```python
from build123d import *

# Parameters (mm, degrees)
SKETCH001_R       = 1.687519
PAD001_DEPTH      = 1.5
SKETCH_R          = 1.746092
PAD_DEPTH         = 2
FUSION_ROLL_ANGLE = 90


with BuildPart() as base_and_horizontal_holder:
    # Sketch001 → Pad001 (new body)
    with BuildSketch(Plane.XZ.offset(1.2525)):
        with BuildLine():
            Line((10.979984, 0), (69.999984, 0))
            Line((69.999984, 0), (69.999984, -21.282469))
            ThreePointArc((66.378106, -24.904346), (68.93916, -23.843523), (69.999984, -21.282469))
            Line((22.859289, -24.904346), (66.378106, -24.904346))
            ThreePointArc((10.979984, -13.025041), (14.459352, -21.424978), (22.859289, -24.904346))
            Line((10.979984, 0), (10.979984, -13.025041))
        make_face()
        with Locations((67.250752, -3.727469)):
            Circle(SKETCH001_R, mode=Mode.SUBTRACT)
        with Locations((16.457752, -18.999969)):
            Circle(SKETCH001_R, mode=Mode.SUBTRACT)
    extrude(amount=-PAD001_DEPTH)


with BuildPart() as obj1:
    # Sketch → Pad (new body)
    with BuildSketch(Plane.XY):
        with BuildLine():
            Line((11.012519, -1.25328), (11.012519, 6.997142))
            ThreePointArc((13.001287, 8.992943), (11.59459, 8.405902), (11.012519, 6.997142))
            Line((13.001287, 8.992943), (15, 9))
            ThreePointArc((16.997615, 7.009425), (16.412099, 8.419465), (15, 9))
            Line((16.997615, 7.009425), (16.997615, 4))
            ThreePointArc((16.997615, 4), (17.290509, 3.292893), (17.997615, 3))
            Line((17.997615, 3), (62, 3))
            Line((62, 3), (62.401287, 3))
            ThreePointArc((62.401287, 3), (64.238855, 3.761145), (65, 5.598713))
            Line((65, 5.598713), (65, 6))
            Line((65, 6), (62, 10))
            ThreePointArc((65, 13), (62.87868, 12.12132), (62, 10))
            Line((65, 13), (67, 13))
            ThreePointArc((70, 10), (69.12132, 12.12132), (67, 13))
            Line((70, 10), (70, -1.25328))
            Line((11.012519, -1.25328), (70, -1.25328))
        make_face()
        with Locations((13.988471, 5.299093)):
            Circle(SKETCH_R, mode=Mode.SUBTRACT)
        with Locations((66.082271, 10.342403)):
            Circle(SKETCH_R, mode=Mode.SUBTRACT)
    extrude(amount=PAD_DEPTH)

    # Fusion: union base_and_horizontal_holder
    add(base_and_horizontal_holder.part)


with BuildPart() as obj1_1:
    # Fusion roll: moved
    add(obj1.part.rotate(Axis((0, 0, 0), (1, 0, 0)), FUSION_ROLL_ANGLE))


with BuildPart() as obj1_2:
    # Fusion placement: moved
    add(obj1_1.part.moved(Location((-10.98, 2, 1.25))))


solid = obj1_2.part
```
Input: part model. Units: mm. Frame: model coordinates. A direction names the side the tool comes from. Coordinates: 2 decimals unless noted, no trailing zeros. Write each loop counter-clockwise with the first axis right and the second up, starting at its lowest first coordinate (ties: lowest second). Pieces come first, ordered by that corner, then holes. Notation, with made-up numbers: (26, 86) -> (44, 86) arc R12 cw to (44, 92) -> close; hole circle Ø2 at (49.25, -39.5). An arc over 180 degrees is marked (long way). Answer as a JSON object with one key per item and string values.
1. Access query for faces 1 (the face through (55, 1, 14.25)), 2 (the face through (5.4, 1, 9.7)). Directions: +Z, -Z, +X, -X, +Y, -Y. A direction counts if a zero-diameter tool reaches every point of the face in a straight line with its end or side. Return the directions, or none.
Result set:
{"face 1": "+Z, +X, -X, +Y, -Y", "face 2": "+Z, +Y, -Y"}
2. First-contact query: P1, Ø1.6, axis at y = 1.5, z = 4, coming from the -X side; P2, Ø1.5, axis at y = 4, z = 3, coming from the -X side; P3, Ø1.6, axis at x = 35.5, y = 1, coming from the +Z side; P4, Ø6, axis at x = 52.5, z = 8.5, coming from the -Y side. Flat tips, straight axial feed; report the tip coordinate or a pass-through.
Result set:
{"P1": "stops at x = 0.03", "P2": "passes through", "P3": "stops at z = 4.25", "P4": "stops at y = 0"}
3. Mould query, pull axis X, two halves, no side actions, for faces 3 (the face through (4.674, 1.014, 7.074)), 4 (the face through (29, 1, 4.25)), 5 (the face through (0.63, 1.01, 9.67)), 6 (the face through (59.02, 1, 6)). Classes: released by +X, released by -X, zero draft, split by the parting line, or undercut.
Result set:
{"face 3": "undercut", "face 4": "undercut", "face 5": "released by -X", "face 6": "released by +X"}
4. Material intervals for line 1 (Y direction, x = 56.5, z = 2.5); line 2 (Z direction, x = 25, y = 7.75), sorted ascending. Write a range as from..to.
Result set:
{"line 1": "y = 0..2", "line 2": "z = 0..1.5"}
5. Section A-A on y = 20. Return the cut outline in (x, z), then the cut area to 3 significant figures.
Result set:
{"outline": "(1.09, 0) -> (4.12, 0) -> (4.12, 1.5) -> (1.09, 1.5) -> close; (6.84, 0) -> (59.02, 0) -> (59.02, 1.5) -> (6.84, 1.5) -> close", "area": "82.8 mm2"}
6. Section C-C on z = 9.25. Return the cut outline in (x, y), then the cut area to 3 significant figures.
Result set:
{"outline": "(0.3, 0) -> (5.75, 0) -> (5.75, 2) -> (0.3, 2) -> close; (52.52, 0) -> (59.02, 0) -> (59.02, 2) -> (52.52, 2) -> close", "area": "23.9 mm2"}
